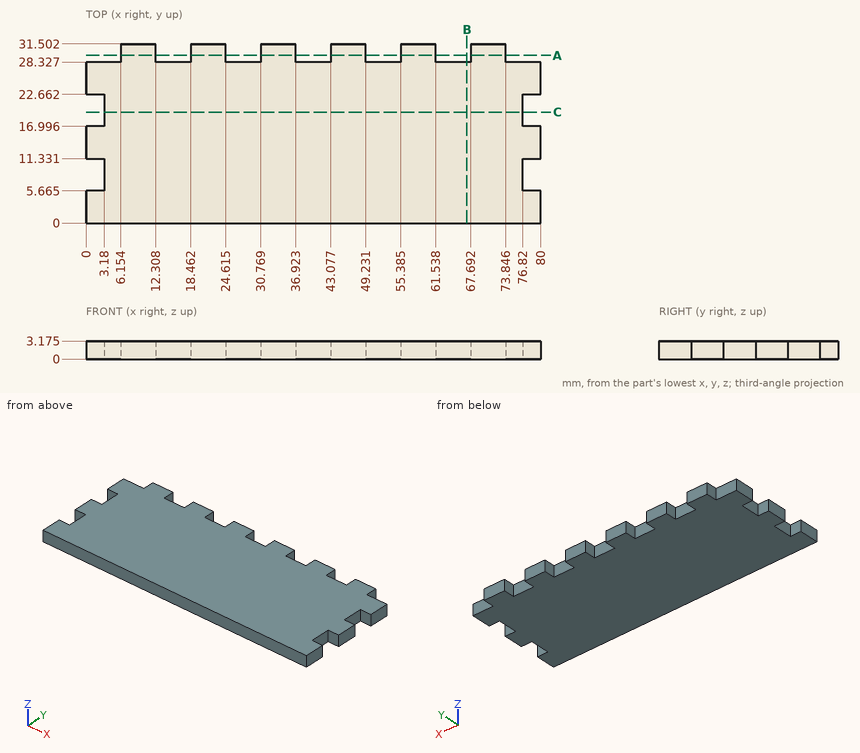
Print and shaded views of the part. All mm, measured from the part's lowest x, y and z. Give positions to 0.01 mm unless a question says otherwise; leave off trailing zeros. Loops run counter-clockwise (first coordinate to the right, second up) from the corner with the lowest first, then second, coordinate; pieces in that order, holes last. Notation, with made-up numbers: (29, 23) -> (55, 23) arc R20 ccw to (55, 38) -> close; hole circle Ø2 at (-32, 3.25). An arc over 180 degrees is marked (long way). Use a Markdown table: item, result.
1. Wall check: L1, parallel to X at y = 29, z = 0.3 (1 decimal); L2, parallel to X at y = 22, z = 1.05; L3, parallel to Y at x = 13, z = 2.4. Give the ranges that are in metal, low to high. Write a range as [from, to].
Check result:
| item | result |
|---|---|
| L1 | x = [6.2, 12.3], [18.5, 24.6], [30.8, 36.9], [43.1, 49.2], [55.4, 61.5], [67.7, 73.8] |
| L2 | x = [3.18, 76.82] |
| L3 | y = [0, 28.33] |
2. Slice it at A-A (y = 29.5). List the corners of the cut face in (x, z) (1 decimal), plus the area to 3 significant figures.
Check result:
| item | result |
|---|---|
| outline | (6.2, 0) -> (12.3, 0) -> (12.3, 3.2) -> (6.2, 3.2) -> close; (18.5, 0) -> (24.6, 0) -> (24.6, 3.2) -> (18.5, 3.2) -> close; (30.8, 0) -> (36.9, 0) -> (36.9, 3.2) -> (30.8, 3.2) -> close; (43.1, 0) -> (49.2, 0) -> (49.2, 3.2) -> (43.1, 3.2) -> close; (55.4, 0) -> (61.5, 0) -> (61.5, 3.2) -> (55.4, 3.2) -> close; (67.7, 0) -> (73.8, 0) -> (73.8, 3.2) -> (67.7, 3.2) -> close |
| area | 117 mm^2 |
3. Flat gauge pins, fed straight in: pin 1 (1.6 mm diameter, centred on y = 30, z = 1, fed in from +X); pin 2 (1.6 mm diameter, centred on y = 30, z = 1.5, fed in from -X); pin 3 (1 mm diameter, centred on x = 28, z = 1, fed in from +Y). Where does each tip first touch, or does it go through?
Check result:
| item | result |
|---|---|
| pin 1 | stops at x = 73.85 |
| pin 2 | stops at x = 6.15 |
| pin 3 | stops at y = 28.33 |
4. Slice it at C-C (y = 19.5). List the corners of the cut face in (x, z) (1 decimal).
Check result:
| item | result |
|---|---|
| outline | (3.2, 0) -> (76.8, 0) -> (76.8, 3.2) -> (3.2, 3.2) -> close |
5. Slice it at B-B (x = 67). List the corners of the cut face in (y, z) (1 decimal).
Check result:
| item | result |
|---|---|
| outline | (0, 0) -> (28.3, 0) -> (28.3, 3.2) -> (0, 3.2) -> close |
